Autodesk Inventor part; units mm, degrees
ref_plane "YZ Plane" through (0, 0, 0) normal (1, 0, 0) x (0, 1, 0)
ref_plane "XZ Plane" through (0, 0, 0) normal (0, 1, 0) x (-1, 0, 0)
ref_plane "XY Plane" through (0, 0, 0) normal (0, 0, 1) x (1, 0, 0)
sketch "Skizze1" plane through (0, 0, 0) normal (0, 0, 1) x (1, 0, 0)
  line L0 (-15, -15) -> (15, -15)
  line L1 (15, -15) -> (15, 15)
  line L2 (15, 15) -> (-15, 15)
  line L3 (-15, 15) -> (-15, -15)
  line L4 (-15, -15) -> (15, 15) construction
  line L5 (15, -15) -> (-15, 15) construction
  point P0 (0, 0)
  dimension "d0" = 30
  dimension "d1" = 30
extrude "Extrusion1" add sketch "Skizze1" along normal blind 100
sketch "Skizze2" plane through (0, 0, 0) normal (0, 0, -1) x (-1, 0, 0)
  circle A0 centre (40, -40) radius 7.5
  circle A1 centre (-40, -40) radius 7.5
  circle A2 centre (-40, 40) radius 7.5
  circle A3 centre (40, 40) radius 7.5
  line L0 (0, -66.5) -> (0, 66.5)
  line L1 (66.5, 0) -> (-66.5, 0)
  line L2 (45.6471, -35.0643) -> (15, 0)
  line L3 (15, 15) -> (15, -15)
  line L4 (35.8038, -46.2162) -> (0, -15)
  line L5 (15, -15) -> (-15, -15)
  line L6 (0, -15) -> (-35.0643, -45.6471)
  line L7 (-15, -15) -> (-15, 15)
  line L8 (-15, 0) -> (-46.2162, -35.8038)
  line L9 (-15, 15) -> (15, 15)
  line L10 (0, 15) -> (-34.4135, 45.0041)
  line L11 (-15, 0) -> (-45.6471, 35.0643)
  line L12 (0, 15) -> (35.0643, 45.6471)
  line L13 (15, 0) -> (45.0041, 34.4135)
  point P0 (0, 0)
  dimension "d4" = 15
  dimension "d5" = 15
  dimension "d6" = 15
  dimension "d7" = 15
  dimension "d8" = 40
  dimension "d9" = 40
extrude "Extrusion2" add sketch "Skizze2" along normal blind 10 contours A0 L4 | A0 L4 L5 L3 L2 | L3 L5 L0 L1 | L1 L0 L9 L3 | L3 L9 L12 A3 L13 | L5 L7 L1 L0 | L6 A1 L8 L7 L5 | L1 L7 L9 L0 | A3 | A1 L8 | L9 L7 L11 A2 L10 | A2 picked at (40.9311, -37.6896) picked at (-39.2767, -42.7034)
sketch "Skizze3" plane through (0, 0, -10) normal (0, 0, -1) x (-1, 0, 0)
  arc A0 (45.0041, 34.4135) -> (35.0643, 45.6471) centre (40, 40) ccw
  circle A1 centre (40, 40) radius 7.5
  arc A2 (35.8038, -46.2162) -> (45.6471, -35.0643) centre (40, -40) ccw
  circle A3 centre (40, -40) radius 7.5
  arc A4 (-46.2162, -35.8038) -> (-35.0643, -45.6471) centre (-40, -40) ccw
  circle A5 centre (-40, -40) radius 7.5
  arc A6 (-34.4135, 45.0041) -> (-45.6471, 35.0643) centre (-40, 40) ccw
  circle A7 centre (-40, 40) radius 7.5
  point P0 (0, 0)
  point P1 (-45.6471, 35.0643)
  point P2 (-34.4135, 45.0041)
  point P3 (45.6471, -35.0643)
  point P4 (-35.0643, -45.6471)
  point P5 (-46.2162, -35.8038)
  point P6 (35.0643, 45.6471)
extrude "Extrusion3" add sketch "Skizze3" along normal blind 10
sketch "Skizze4" plane through (-15, 15, 100) normal (0, 1, 0) x (1, 0, 0)
  circle A0 centre (15, 20) radius 12.5
  line L0 (30, 0) -> (0, 0)
  point P0 (15, 100)
  dimension "d14" = 25
  dimension "d15" = 20
extrude "Extrusion4" cut sketch "Skizze4" against normal blind 5
sketch "Skizze5" plane through (0, 10, 80) normal (0, 1, 0) x (1, 0, 0)
  circle A0 centre (0, 0) radius 7.5
  point P0 (0, 80)
  dimension "d18" = 15
extrude "Extrusion5" add sketch "Skizze5" along normal blind 10
fillet "Rundung1" radius 10 2 edges at (15, 0, 100) (-15, 0, 100)
fillet "Rundung2" radius 10 5 edges at (12.0711, -15, 97.0711) (0, -15, 100) (-12.0711, -15, 97.0711) (-15, -15, 45) (15, -15, 45)
chamfer "Fase3" distance 2 angle 45 3 edges at (-7.5, 20, 80) (-7.5, 10, 80) (-12.5, 10, 80)
fillet "Rundung3" radius 2 5 edges at (12.0711, 15, 97.0711) (0, 15, 100) (-12.0711, 15, 97.0711) (-15, 15, 45) (15, 15, 45)
fillet "Rundung4" radius 10 4 edges at (0, -15, -5) (15, 0, -5) (-15, 0, -5) (0, 15, -5)
equation "\"d5\" = d4"
equation "\"d6\" = d4"
equation "\"d7\" = d4"
equation "\"d9\" = d8"
properties part number "Sensor"
Input: part model. Units: mm. Frame: model coordinates. A direction names the side the tool comes from. Round coordinates to 2 decimals unless told otherwise and drop trailing zeros. Write each loop counter-clockwise with the first axis right and the second up, starting at its lowest first coordinate (ties: lowest second). Pieces come first, ordered by that corner, then holes. Notation, with made-up numbers: (-3, 65.25) -> (8, 65.25) arc R30 ccw to (8, 104.25) -> close; hole circle Ø10 at (-8.5, 1.5). An arc over 180 degrees is marked (long way). Answer as CSV lines item,"result".
1. Reachability of faces 1 (the cylindrical face through (-34.26, -35.17, -14.93)), 2 (the flat face through (33.02, 20.62, -4.93)), 3 (the flat face through (-20.62, 33.02, -4.93)), 4 (the flat face through (-21.396, -33.655, -4.93)) from +Z, -Z, +X, -X, +Y, -Y: full face, straight path, thin tool, end or side. Return the list, or none.
Geometry says:
face 1,"-Z"
face 2,"+Z, -Z, +X"
face 3,"+Z, -Z, +Y"
face 4,"+Z, -Z, -Y"
2. Section A-A (x = -28). Return the cut outline in (y, z).
Geometry says:
outline,"(-39.41, -10) -> (-14.87, -10) -> (-14.87, 0) -> (-39.41, 0) -> close; (14.91, -10) -> (39.47, -10) -> (39.47, 0) -> (14.91, 0) -> close"
3. Contact query for flat-ended pins moving along their axis: P1, Ø9, axis at x = 2.5, z = 81.5, coming from the +Y side; P2, Ø1.3, axis at x = 45.5, y = -35.5, coming from the +Z side; P3, Ø20, axis at y = 4.5, z = 63.5, coming from the -X side. Output: stop coordinate, or through.
Geometry says:
P1,"stops at y = 20"
P2,"stops at z = 0"
P3,"stops at x = -15"
4. Section D-D (x = 40). Return the cut outline in (y, z), plus the area to 3 significant figures.
Geometry says:
outline,"(-47.5, -20) -> (-32.5, -20) -> (-32.5, -10) -> (-28.67, -10) -> (-28.67, 0) -> (-47.5, 0) -> close; (28.6, -10) -> (32.5, -10) -> (32.5, -20) -> (47.5, -20) -> (47.5, 0) -> (28.6, 0) -> close"
area,"677 mm^2"
5. Section B-B (y = -25). Return the cut outline in (x, z).
Geometry says:
outline,"(-36.85, -10) -> (-11.47, -10) -> (-11.47, 0) -> (-36.85, 0) -> close; (11.44, -10) -> (36.8, -10) -> (36.8, 0) -> (11.44, 0) -> close"
6. Mould query, pull axis Y, two halves, no side actions, for faces 5 (the cylindrical face through (11.99, 4.13, 97.15)), 6 (the cylindrical face through (0.07, -11.99, 97.15)), 7 (the flat face through (-33.37, -21.02, -4.93)). Classes: +Y half, -Y half, draft (parallel to the pull), parting line (faces both ways), or undercut.
Geometry says:
face 5,"draft"
face 6,"-Y half"
face 7,"undercut"
7. Section C-C (z = 55). Return the cut outline in (x, y).
Geometry says:
outline,"(-15, -5) arc R10 ccw to (-5, -15) -> (5, -15) arc R10 ccw to (15, -5) -> (15, 13) arc R2 ccw to (13, 15) -> (-13, 15) arc R2 ccw to (-15, 13) -> close"
8. Ray query, L1, parallel to X at y = 13, z = 80; L2, parallel to Z at x = 0, y = 13; L3, parallel to Z at x = 0, y = 14.25. Return the intervals inside material, ascending. Write a range as [from, to].
Geometry says:
L1,"x = [-15, -12.5], [-7.5, 7.5], [12.5, 15]"
L2,"z = [-10, 67.5], [72.5, 87.5], [92.5, 100]"
L3,"z = [-10, 67.5], [72.5, 87.5], [92.5, 99.56]"
